```python
from build123d import *

# Parameters (mm, degrees)
BOSS_EXTRUDE1_DEPTH      = 15
BOSS_EXTRUDE1_DEPTH_BACK = 15
SKETCH1_R                = 125
SKETCH2_R                = 25
BOSS_EXTRUDE2_DEPTH      = 20
SKETCH3_R                = 2.5
BOSS_EXTRUDE3_DEPTH      = 15
CIRPATTERN1_COUNT        = 4


with BuildPart() as part:
    # Sketch1 → Boss-Extrude1 (new, two sides: drawn at the far end of the back side and taken through both)
    with BuildSketch(Plane.XY.offset(-BOSS_EXTRUDE1_DEPTH_BACK)):
        with Locations((-0.2079628, -0.516116692)):
            Circle(SKETCH1_R)
        Polygon((-30, 430), (30, 430), (30, 30), (430, 30), (430, -30), (30, -30), (30, -430), (-30, -430), (-30, -30), (-430, -30), (-430, 30), (-30, 30), align=None)
    extrude(amount=BOSS_EXTRUDE1_DEPTH + BOSS_EXTRUDE1_DEPTH_BACK)

    # Sketch2 → Boss-Extrude2 (add)
    with BuildSketch(Plane.XY.offset(15)):
        with Locations((390, 0)):
            Circle(SKETCH2_R)
    boss_extrude2 = extrude(amount=BOSS_EXTRUDE2_DEPTH)

    # Sketch3 → Boss-Extrude3 (add)
    with BuildSketch(Plane.XY.offset(35)):
        with Locations((390, 0)):
            Circle(SKETCH3_R)
    boss_extrude3 = extrude(amount=BOSS_EXTRUDE3_DEPTH)

    # CirPattern1: Boss-Extrude2, Boss-Extrude3 ×4 about axis
    cirpattern1_axis = Axis((-0.2079628, -0.516116692, 0), (0, 0, 1))
    add([boss_extrude2.rotate(cirpattern1_axis, i * 360 / CIRPATTERN1_COUNT) for i in range(1, CIRPATTERN1_COUNT)])
    add([boss_extrude3.rotate(cirpattern1_axis, i * 360 / CIRPATTERN1_COUNT) for i in range(1, CIRPATTERN1_COUNT)])


solid = part.part
```
Input: part model. Units: mm. Frame: model coordinates. A direction names the side the tool comes from. Coordinates: 2 decimals unless noted, no trailing zeros. Write each loop counter-clockwise with the first axis right and the second up, starting at its lowest first coordinate (ties: lowest second). Pieces come first, ordered by that corner, then holes. Notation, with made-up numbers: M 55,-8 L 105,-8 A14 cw 105,-4 Z; hole C 74,39 d1. An arc over 180 degrees is marked long. Use one line per item in the form item = value.
Q1. Draft query along X for faces 1 (the face through (278, -30, 0)), 2 (the face through (30, -274, 0)), 3 (the face through (-370.577, 14.18, 24.86)). Return one class per face: released by +X, released by -X, zero draft, split by the parting line, or undercut.
Answer below:
face_1 = zero draft
face_2 = released by +X
face_3 = undercut
Q2. Material intervals for probe 1 along Y at (x, z) = (162, 9.5); probe 2 along Y at (x, z) = (390.5, 39.5), sorted ascending. Write a range as from..to.
Answer below:
probe_1 = -30..30
probe_2 = -2.45..2.45
Q3. First-contact query: pin 1 (15 mm diameter, centred on y = -347, z = 1, fed in from -X); pin 2 (15 mm diameter, centred on x = 7, y = 400.5, fed in from +Z); pin 3 (2 mm diameter, centred on x = 82.5, z = -4.5, fed in from -Y). Flat tips, straight axial feed; report the tip coordinate or a pass-through.
Answer below:
pin_1 = -30
pin_2 = 35
pin_3 = -95.11
Q4. Section B-B (y = -333). Return loops of the section in (x, z), plus the area to 3 significant figures.
Answer below:
outline = M -30,-15 L 30,-15 L 30,15 L -30,15 Z
area = 1,800 mm²
Q5. Section A-A (z = 3.5). Return loops of the section in (x, y).
Answer below:
outline = M -430,-30 L -121.68,-30 A125 ccw -30,-121.91 L -30,-430 L 30,-430 L 30,-121.81 A125 ccw 121.27,-30 L 430,-30 L 430,30 L 121.01,30 A125 ccw 30,120.78 L 30,430 L -30,430 L -30,120.88 A125 ccw -121.43,30 L -430,30 Z
Q6. Set-up query: faces 4 (the face through (273, 30, 0)), 5 (the face through (-30, 273, 0)), 6 (the face through (0, 430, 0)), 7 (the face through (-2, 2, 15)), 8 (the face through (-30, -278, 0)). Return all of +Z, -Z, +X, -X, +Y, -Y with unobstructed straight access to the full face (end or side cutting, diameter ignored); none if empty.
Answer below:
face_4 = +Z, -Z, +X, +Y
face_5 = +Z, -Z, -X, +Y
face_6 = +Z, -Z, +X, -X, +Y
face_7 = +Z
face_8 = +Z, -Z, -X, -Y
